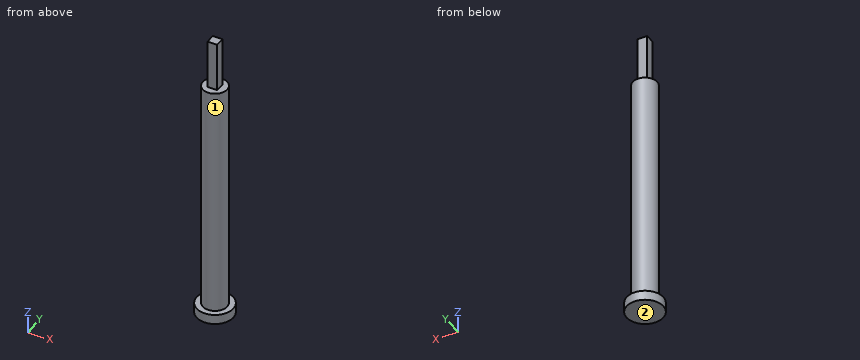
from build123d import *

# Parameters (mm, degrees)
F0_R     = 7.5
F1_DEPTH = 4
F2_R     = 5
F3_DEPTH = 100
F4_W     = 4
F4_H     = 4
F5_DEPTH = 20


with BuildPart() as f1:
    # F0 (on Top) → F1 (new body)
    with BuildSketch(Plane.XY):
        Circle(F0_R)
    extrude(amount=F1_DEPTH)

    # F2 (on Top) → F3 (join)
    with BuildSketch(Plane.XY):
        Circle(F2_R)
    extrude(amount=F3_DEPTH)

    # F4 (on face) → F5 (join)
    with BuildSketch(Plane.XY.offset(100)):
        Rectangle(F4_W, F4_H)
    extrude(amount=F5_DEPTH)


solid = f1.part
CAD build for the part. Positions are in the model's coordinates, mm. Face numbers are marked on the shaded views. A direction names the side the tool comes from. Round coordinates to 2 decimals unless told otherwise and drop trailing zeros. Write each loop counter-clockwise with the first axis right and the second up, starting at its lowest first coordinate (ties: lowest second). Pieces come first, ordered by that corner, then holes.
(1) Drop flat-ended pins along their axis: P1, Ø2, axis at y = -1, z = 108, coming from the +X side; P2, Ø8, axis at y = -5.5, z = 29, coming from the +X side; P3, Ø1.2, axis at x = -0.5, z = 107.5, coming from the +Y side. Give the stop position or say it passes through.
(2) Slice it at A-A, the plane x = 0. Write the cut outline in (y, z).
(3) Slice it at C-C, the plane z = 92.5. Write the cut outline in (x, y), and give its area (3 significant figures).
(4) 3-axis set-ups, long thin cutter, end or side, ignore diameter. For the marked faces 1 and 2: which of +Z, -Z, +X, -X, +Y, -Y reach the whole face in a straight line?
(5) Probe line 1 along Z through (x, y) = (1.5, 3.25); line 2 along Z through (x, y) = (5.75, -4.5); line 3 along Y through (x, z) = (0.25, 39). List the from-to ranges inside material, lowest first.
(6) Slice it at D-D, the plane x = 6. Write the cut outline in (y, z).
From the geometry:
1. P1: stops at x = 2
1. P2: stops at x = 4.77
1. P3: stops at y = 2
2. outline: (-7.5, 0) - (7.5, 0) - (7.5, 4) - (5, 4) - (5, 100) - (2, 100) - (2, 120) - (-2, 120) - (-2, 100) - (-5, 100) - (-5, 4) - (-7.5, 4) - close
3. outline: circle Ø10 at (0, 0)
3. area: 78.5 mm2
4. face 1: +Z
4. face 2: -Z, +X, -X, +Y, -Y
5. line 1: z = 0 to 100
5. line 2: z = 0 to 4
5. line 3: y = -4.99 to 4.99
6. outline: (-4.5, 0) - (4.5, 0) - (4.5, 4) - (-4.5, 4) - close
